Autodesk Inventor part; units mm, degrees
ref_plane "YZ Plane" through (0, 0, 0) normal (1, 0, 0) x (0, 1, 0)
ref_plane "XZ Plane" through (0, 0, 0) normal (0, 1, 0) x (-1, 0, 0)
ref_plane "XY Plane" through (0, 0, 0) normal (0, 0, 1) x (1, 0, 0)
sketch "Эскиз5" plane through (0, 0, 0) normal (0, 0, 1) x (1, 0, 0)
  line L0 (0, 0) -> (20, 0)
  line L1 (20, 0) -> (20, 25)
  line L2 (16, 29) -> (4, 29)
  line L3 (0, 25) -> (0, 0)
  line L4 (4, 29) -> (0, 25)
  line L5 (16, 29) -> (20, 25)
  point P0 (20, 29)
  point P1 (0, 29)
  dimension "d33" = 20
  dimension "d34" = 29
  dimension "d35" = 4
  dimension "d36" = 4
  dimension "d37" = 4
  dimension "d38" = 4
revolve "Вращение3" add sketch "Эскиз5" angle 360 about axis through (0, 0, 0) along (1, 0, 0)
sketch "Эскиз6" plane through (0, 0, 0) normal (-1, 0, 0) x (0, 0, 1)
  line L0 (0, 0) -> (0, 23) construction
  dimension "d40" = 23
hole "Отверстие3" at (0, 23, 0) direction (1, 0, 0) diameter 4 depth 4 tip angle 150
sketch "Эскиз7" plane through (20, 0, 0) normal (1, 0, 0) x (0, 0, -1)
  point P0 (0, 0)
  point P1 (0, 0)
hole "Отверстие4" at (20, 0, 0) direction (-1, 0, 0) diameter 12 depth 6 countersink diameter 14 countersink angle 82
sketch "Эскиз8" plane through (14, 0, 0) normal (1, 0, 0) x (0, 0, -1)
  circle A0 centre (0, 0) radius 7
  dimension "d55" = 14
extrude "Выдавливание1" cut sketch "Эскиз8" against normal blind 0.5
thread "Резьба4"
properties part number "711132"
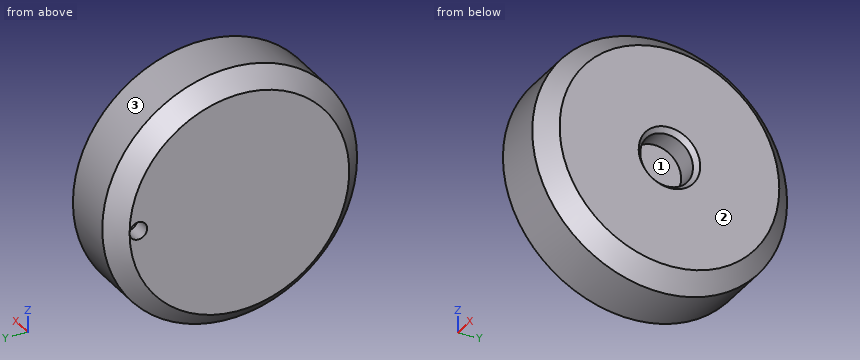
The model under review builds one solid part; all positions refer to its coordinate system, in mm. Face numbers are marked on the shaded views. Round coordinates to 2 decimals unless told otherwise and drop trailing zeros. Loops run counter-clockwise (first coordinate to the right, second up) from the corner with the lowest first, then second, coordinate; pieces in that order, holes last. Notation, with made-up numbers: (75.25, 52.25) -> (89.25, 52.25) arc R31 ccw to (89.25, 91.25) -> close; hole circle Ø2 at (-0.5, 21.25). An arc over 180 degrees is marked (long way). Answer as a JSON object with one key per item and string values. Group by question number.
1) We need section A-A on y = 0. Write out the cut boundary in (x, z), then the cut area to 3 significant figures.
2) Mouldability with a two-part tool opening along Z and no side actions: class the marked faces 1, 2 and 3 as released by +Z, released by -Z, zero draft, split by the parting line, or undercut.
3) We need section B-B on x = 7.25. Write out the cut boundary in (y, z).
4) For line 1 (Z direction, x = 15.55, y = 0); line 2 (Y direction, x = 2.75, z = 0); line 3 (Y direction, x = 1.65, z = 0), list the stretches that pass through material, from the lowest coordinate up. Write a range as [from, to].
5) For pin 1 Ø1.5 at (x, z) = (17.5, 22) entering from -Y; pin 2 Ø1.5 at (x, y) = (12, -17.5) entering from +Z; pin 3 Ø3 at (x, z) = (10, 4.5) entering from +Y, all flat-tipped, find the tip position at first contact; note any pin that passes through.
Result set:
{
 "1": {"outline": "(0, -25) -> (4, -29) -> (16, -29) -> (20, -25) -> (20, -7) -> (18.85, -6) -> (14, -6) -> (14, -7) -> (13.5, -7) -> (13.5, 7) -> (14, 7) -> (14, 6) -> (18.85, 6) -> (20, 7) -> (20, 25) -> (16, 29) -> (4, 29) -> (0, 25) -> close", "area": "1,050 mm²"},
 "2": {"face 1": "undercut", "face 2": "zero draft", "face 3": "split by the parting line"},
 "3": {"outline": "circle Ø58 at (0, 0)"},
 "4": {"line 1": "[-29, -6], [6, 29]", "line 2": "[-27.75, 21], [25, 27.75]", "line 3": "[-26.65, 21], [25, 26.65]"},
 "5": {"pin 1": "y = -18.03", "pin 2": "z = 23.67", "pin 3": "y = 28.84"}
}
